```python
from build123d import *

# Parameters (mm, degrees)
SKETCH1_R                      = 63.5
SKETCH1_R_2                    = 55.372
BOSS_EXTRUDE1_DEPTH            = 3.175
BOSS_EXTRUDE2_DEPTH            = 3.175
SKETCH37_R                     = 0.889
CUT_EXTRUDE19_DEPTH            = 116.700962847
DRAFT20_ANGLE                  = 2
DRAFT21_ANGLE                  = 2
CIRPATTERN7_COUNT              = 7
DRAFT21_OF_CIRPATTERN7_2_ANGLE = 2
DRAFT21_OF_CIRPATTERN7_3_ANGLE = 2
DRAFT21_OF_CIRPATTERN7_4_ANGLE = 2


with BuildPart() as part:
    # Sketch1 → Boss-Extrude1 (new body)
    with BuildSketch(Plane(origin=(0, 0, 0), x_dir=(1, 0, 0), z_dir=(0, 1, 0))):
        with Locations(Location((0, 0, 0), (0, 0, 270))):
            Circle(SKETCH1_R)
        with Locations(Location((0, 0, 0), (0, 0, 270))):
            Circle(SKETCH1_R_2, mode=Mode.SUBTRACT)
    extrude(amount=BOSS_EXTRUDE1_DEPTH)

    # Sketch2 → Boss-Extrude2 (add)
    with BuildSketch(Plane(origin=(0, 0, 0), x_dir=(1, 0, 0), z_dir=(0, 1, 0))):
        with BuildLine():
            ThreePointArc((63.304250692, -4.982152579), (63.5, 0), (63.304250692, 4.982152579))
            ThreePointArc((63.304250692, 4.982152579), (75.956520603, 2.543628775), (88.177394932, 6.627323532))
            ThreePointArc((88.177394932, 6.627323532), (88.826525295, 6.930865115), (89.534602282, 7.04102274))
            ThreePointArc((89.534602282, 7.04102274), (96.666344602, 0), (89.534602282, -7.04102274))
            ThreePointArc((89.534602282, -7.04102274), (88.826525295, -6.930865115), (88.177394932, -6.627323532))
            ThreePointArc((88.177394932, -6.627323532), (75.956520603, -2.543628775), (63.304250692, -4.982152579))
        make_face()
    boss_extrude2 = extrude(amount=BOSS_EXTRUDE2_DEPTH)

    # Sketch37 → Cut-Extrude19 (cut, through all)
    with BuildSketch(Plane(origin=(0, 3.175, 0), x_dir=(1, 0, 0), z_dir=(0, 1, 0))):
        with Locations(Location((89.624744861, 0, 0), (0, 0, 270))):
            Circle(SKETCH37_R)
    cut_extrude19 = extrude(amount=-CUT_EXTRUDE19_DEPTH, mode=Mode.SUBTRACT)

    # Draft20
    draft20_faces = [part.faces().sort_by_distance(p)[0] for p in [
        (0, 1.5875, -55.372),
        (-63.5, 1.5875, 0),
    ]]
    draft(draft20_faces, Plane(origin=(0, 0, 0), x_dir=(0, 0, -1), z_dir=(0, -1, 0)), DRAFT20_ANGLE)

    # Draft21
    draft21_faces = [part.faces().sort_by_distance(p)[0] for p in [
        (88.826525295, 1.5875, 6.930865115),
        (75.956520603, 1.587499999, 2.543628775),
        (88.826525295, 1.5875, -6.930865115),
        (96.666344602, 1.5875, 0),
        (75.956520603, 1.5875, -2.543628775),
    ]]
    draft(draft21_faces, Plane(origin=(0, 0, 0), x_dir=(0, 0, -1), z_dir=(0, -1, 0)), DRAFT21_ANGLE)

    # CirPattern7: Boss-Extrude2, Cut-Extrude19 ×7 about axis, 3 skipped
    cirpattern7_axis = Axis((0, 0, 0), (0, -1, 0))
    add([boss_extrude2.rotate(cirpattern7_axis, i * 360 / CIRPATTERN7_COUNT) for i in range(1, CIRPATTERN7_COUNT) if i not in (2, 4, 6)])
    add([cut_extrude19.rotate(cirpattern7_axis, i * 360 / CIRPATTERN7_COUNT) for i in range(1, CIRPATTERN7_COUNT) if i not in (2, 4, 6)], mode=Mode.SUBTRACT)

    # Draft21 of CirPattern7 2
    draft21_of_cirpattern7_2_faces = [part.faces().sort_by_distance(p)[0] for p in [
        (49.963664108, 1.5875, 73.768697671),
        (45.369426924, 1.587499999, 60.971125707),
        (60.801201204, 1.5875, 65.126050237),
        (60.270480042, 1.5875, 75.576791505),
        (49.346805037, 1.5875, 57.799272505),
    ]]
    draft(draft21_of_cirpattern7_2_faces, Plane(origin=(0, 0, 0), x_dir=(0.7818314824680298, 0, -0.6234898018587336), z_dir=(0, -1, 0)), DRAFT21_OF_CIRPATTERN7_2_ANGLE)

    # Draft21 of CirPattern7 3
    draft21_of_cirpattern7_3_faces = [part.faces().sort_by_distance(p)[0] for p in [
        (-83.037123606, 1.5875, 32.295891232),
        (-69.538099541, 1.587499999, 30.664568831),
        (-77.022744263, 1.5875, 44.784878624),
        (-87.09336706, 1.5875, 41.941955043),
        (-67.330821213, 1.5875, 35.248029508),
    ]]
    draft(draft21_of_cirpattern7_3_faces, Plane(origin=(0, 0, 0), x_dir=(0.43388373911755823, 0, 0.900968867902419), z_dir=(0, -1, 0)), DRAFT21_OF_CIRPATTERN7_3_ANGLE)

    # Draft21 of CirPattern7 4
    draft21_of_cirpattern7_4_faces = [part.faces().sort_by_distance(p)[0] for p in [
        (-13.008667512, 1.5875, -88.141721431),
        (-14.422061213, 1.587499999, -74.618142699),
        (-26.522855225, 1.5875, -85.057196274),
        (-21.510285283, 1.5875, -94.242717521),
        (-19.381770596, 1.5875, -73.486121397),
    ]]
    draft(draft21_of_cirpattern7_4_faces, Plane(origin=(0, 0, 0), x_dir=(-0.9749279121818237, 0, 0.2225209339563137), z_dir=(0, -1, 0)), DRAFT21_OF_CIRPATTERN7_4_ANGLE)


solid = part.part
```
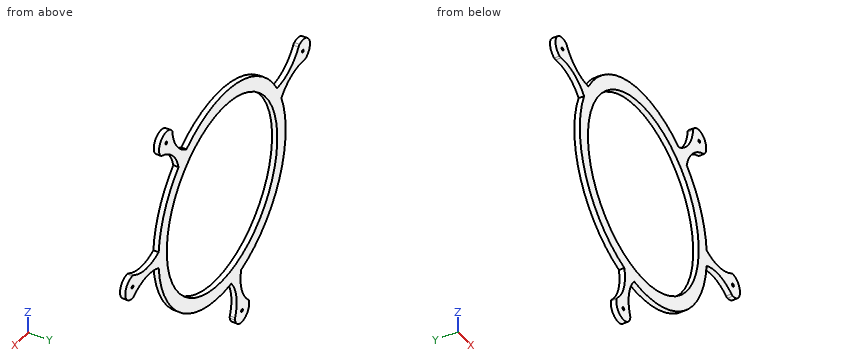
The listing builds one solid part. Answer for the finished solid, in the listing's coordinates (mm). Give positions to 0.01 mm unless a question says otherwise; leave off trailing zeros. Loops run counter-clockwise (first coordinate to the right, second up) from the corner with the lowest first, then second, coordinate; pieces in that order, holes last. Notation, with made-up numbers: (-14.5, 60.5) - (1.5, 60.5) arc R23 ccw to (1.5, 88.5) - close; hole circle Ø6 at (5, 46.25). An arc over 180 degrees is marked (long way). Answer as CSV lines item,"result". Start each with the question number.
Item 1: A cutting plane is placed at B-B on y = 0.85. Count the separate pieces of the cut face and the enclosed holes in it, then the cut area to 3 significant figures.
Item 2: Each of these flat-tipped pins is pushed along its axis until it touches: pin 1 (1.5 mm diameter, centred on y = 0.5, z = -1, fed in from -X); pin 2 (1 mm diameter, centred on y = 1.5, z = -8, fed in from -X). Where does it stop, or does it pass through?
Item 3: Find the intervals of material crossed by line 1 (X direction, y = 1.25, z = 0); line 2 (Z direction, x = 46.5, y = 2.25); line 3 (X direction, y = 0.5, z = 5.5), in increasing order. Write a range as from..to.
Item 4: A cutting plane is placed at A-A on x = 0. Determine the outline of the cut face in (y, z) (3 decimals), then the cut area to 3 significant figures.
Found:
1,separate pieces,"1"
1,enclosed holes,"5"
1,area,"4,160 mm^2"
2,pin 1,"stops at x = -63.54"
2,pin 2,"stops at x = -63.11"
3,line 1,"x = -63.54..-55.33, 55.33..88.74, 90.51..96.71"
3,line 2,"z = -43.36..-29.92, 29.92..43.36, 53.87..62.91"
3,line 3,"x = -63.28..-55.08, 55.08..63.28, 86.24..94.05"
4,outline,"(0, -63.5) - (3.175, -63.611) - (3.175, -55.261) - (0, -55.372) - close; (0, 55.372) - (3.175, 55.261) - (3.175, 63.611) - (0, 63.5) - close"
4,area,"52.3 mm^2"
